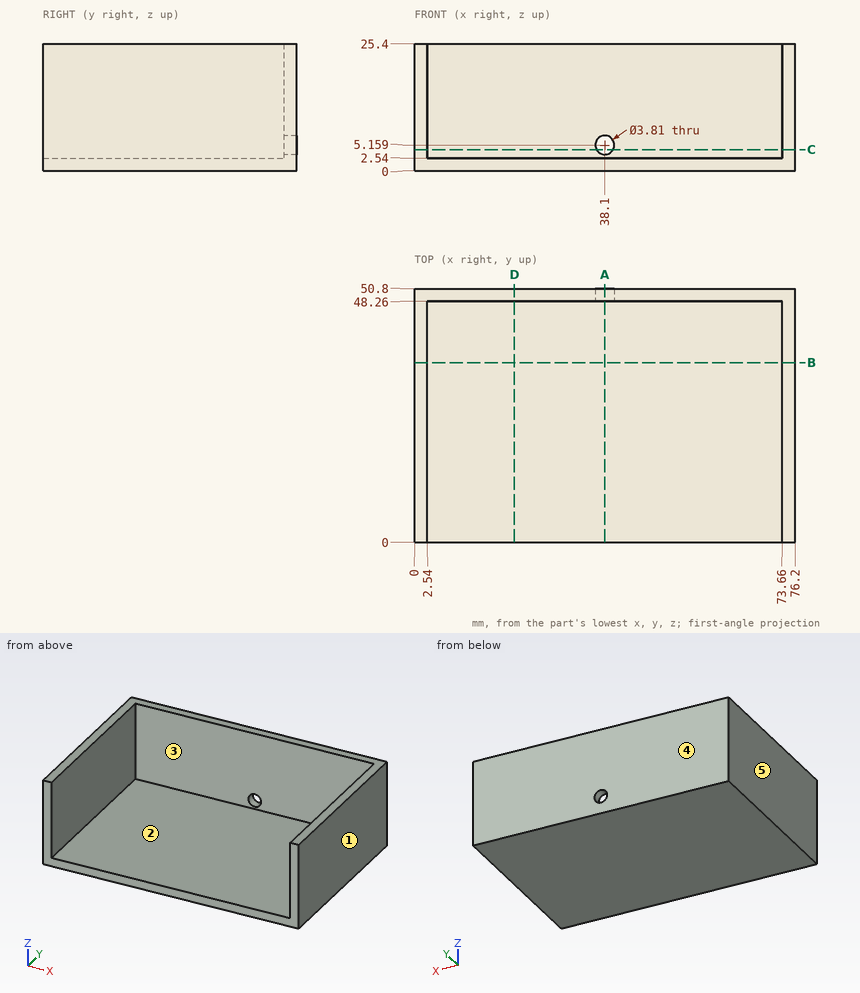
Study the drawing (mm; zero at the part's minimum x, y, z) and answer. A direction names the side the tool comes from. Give positions to 0.01 mm unless a question says otherwise; leave off trailing zeros. Write each loop counter-clockwise with the first axis right and the second up, starting at its lowest first coordinate (ties: lowest second). Pieces come first, ordered by that corner, then holes. Notation, with made-up numbers: (70.25, -27) - (96.25, -27) arc R32 cw to (96.25, 10) - close; hole circle Ø7 at (4, -30.5). An arc over 180 degrees is marked (long way). Write item = value, one per line. Start each with the question number.
Item 1: Find section D-D (x = 20). Give the vertices of the cut face in (y, z).
Item 2: Each of these flat-tipped pins is pushed along its axis until it touches: P1, Ø8, axis at x = 15, y = 31, coming from the -Z side; P2, Ø7, axis at x = 22.5, z = 19.5, coming from the -Y side; P3, Ø24, axis at x = 48, y = 18, coming from the +Z side. Where does it stop, or does it pass through?
Item 3: Find the intervals of material crossed by probe 1 along X at (y, z) = (24, 4.5); probe 2 along Z at (x, y) = (38.1, 48.95); probe 3 along Y at (x, z) = (34, 3.75), in increasing order. Write a range as [from, to].
Item 4: Find section A-A (x = 38.1). Give the vertices of the cut face in (y, z), then the cut area to 3 significant figures.
Item 5: Find section B-B (y = 36). Give the vertices of the cut face in (x, z), then the cut area to 3 significant figures.
Item 6: A tool of negligible diameter and unlimited length cuts with its end or side. For the marked faces 1 and 2, from which of +Z, -Z, +X, -X, +Y, -Y can it reach the whole face along a straight path? Write none if from no direction.
Item 7: The mould has two halves that part along X. Classify the marked faces 3, 4 and 5: +X half, -X half, draft (parallel to the pull), parting line (faces both ways), or undercut.
Item 8: Find section C-C (z = 4.25). Give the vertices of the cut face in (x, y).
Response:
q1.outline = (0, 0) - (50.8, 0) - (50.8, 25.4) - (48.26, 25.4) - (48.26, 2.54) - (0, 2.54) - close
q2.P1 = 0
q2.P2 = 48.26
q2.P3 = 2.54
q3.probe_1 = [0, 2.54], [73.66, 76.2]
q3.probe_2 = [0, 3.25], [7.06, 25.4]
q3.probe_3 = [48.26, 50.8]
q4.outline = (0, 0) - (50.8, 0) - (50.8, 3.25) - (48.26, 3.25) - (48.26, 2.54) - (0, 2.54) - close; (48.26, 7.06) - (50.8, 7.06) - (50.8, 25.4) - (48.26, 25.4) - close
q4.area = 177 mm²
q5.outline = (0, 0) - (76.2, 0) - (76.2, 25.4) - (73.66, 25.4) - (73.66, 2.54) - (2.54, 2.54) - (2.54, 25.4) - (0, 25.4) - close
q5.area = 310 mm²
q6.face_1 = +Z, -Z, +X, +Y, -Y
q6.face_2 = +Z, -Y
q7.face_3 = undercut
q7.face_4 = draft
q7.face_5 = -X half
q8.outline = (0, 0) - (2.54, 0) - (2.54, 48.26) - (36.43, 48.26) - (36.43, 50.8) - (0, 50.8) - close; (39.77, 48.26) - (73.66, 48.26) - (73.66, 0) - (76.2, 0) - (76.2, 50.8) - (39.77, 50.8) - close
